For this review, take the finished solid that the model builds, in its own axes (mm). A direction names the side the tool comes from. Give positions to 0.01 mm unless a question says otherwise; leave off trailing zeros. Write each loop counter-clockwise with the first axis right and the second up, starting at its lowest first coordinate (ties: lowest second). Pieces come first, ordered by that corner, then holes. Notation, with made-up numbers: M 53,-37 L 76,-37 A34 ccw 76,2 Z; hole C 78.5,68 d10. An arc over 180 degrees is marked long. Use one line per item in the form item = value. Start each with the question number.
Q1. For probe 1 along Y at (x, z) = (-15.5, -8.25); probe 2 along Z at (x, y) = (26.75, -45); probe 3 along Y at (x, z) = (29.5, -11.5), list the stretches that pass through material, from the lowest coordinate up. Write a range as [from, to].
Q2. Consider section D-D on y = 30. Write out the cut boundary in (x, z), and give its area (3 significant figures).
Q3. Clearance check with flat-ended pins moving along their axes: pin 1 Ø3.5 at (y, z) = (-46, -7) entering from +X; pin 2 Ø3.5 at (y, z) = (39.5, -16.5) entering from -X; pin 3 Ø1 at (y, z) = (40.5, -16.5) entering from -X; pin 4 Ø6 at (x, z) = (-49, -12) entering from +Y. State where each tip first meets the part, or that it passes through.
Q4. Tool access review of faces 4 (the cylindrical face through (16.39, 41.39, -6.41)), 5 (the cylindrical face through (30.886, 47.003, -7.369)), 6 (the flat face through (-71.2, 9.44, -15.46)), 7 (the flat face through (-14, -1, -13)), 8 (the cylindrical face through (25.505, 0.22, -6.409)): name each direction out of +Z, -Z, +X, -X, +Y, -Y from which nothing blocks a thin tool from reaching the whole face with its end or side.
Q5. Mouldability with a two-part tool opening along X and no side actions: class faces 1 (the flat face through (21, -45, -8)), 2 (the flat face through (-18.25, 0, -16)), 3 (the cylindrical face through (30.886, 8.452, -6.581)) as released by +X, released by -X, zero draft, split by the parting line, or undercut.
Q6. Consider section A-A on x = 30.5. Give the number of separate pieces and of enclosed holes in the cut face, and give its area (3 significant figures).
Q7. Consider section B-B on x = -30.5. Write out the cut boundary in (y, z), and give its area (4 significant figures).
```python
from build123d import *

# Parameters (mm, degrees)
PAD_DEPTH       = 50
POCKET_DEPTH    = 18.001
SKETCH003_R     = 10.6
POCKET001_DEPTH = 30.4
SKETCH004_R     = 10.6
POCKET002_DEPTH = 30.4
SKETCH005_R     = 1.65
SKETCH005_R_2   = 2.65
POCKET007_DEPTH = 18.001
POCKET008_DEPTH = 5
SKETCH006_R     = 2.65
POCKET009_DEPTH = 18.001
SKETCH007_R     = 5
POCKET010_DEPTH = 13
SKETCH008_R     = 2.1
POCKET011_DEPTH = 20


with BuildPart() as part:
    # Sketch001 → Pad (new body, symmetric)
    with BuildSketch(Plane.XZ):
        with BuildLine():
            Line((-20.5, 0), (-6.5, 0))
            ThreePointArc((-6.5, 0), (0, -6.5), (6.5, 0))
            Line((6.5, 0), (20.5, 0))
            Line((20.5, 0), (40.5, 0))
            Line((40.5, 0), (40.5, -18))
            Line((40.5, -18), (20.5, -18))
            Line((20.5, -18), (-120.5, -18))
            Line((-120.5, -18), (-120.5, -13))
            Line((-20.5, -13), (-120.5, -13))
            Line((-20.5, 0), (-20.5, -13))
        make_face()
    extrude(amount=PAD_DEPTH, both=True)

    # Sketch002 → Pocket (cut, through all)
    with BuildSketch(Plane.XY):
        Polygon((-20.5, 50), (-120.5, 50), (-120.5, -30), align=None)
    extrude(amount=-POCKET_DEPTH, mode=Mode.SUBTRACT)

    # Sketch003 (on DatumPlane) → Pocket001 (cut)
    with BuildSketch(Plane.XZ.offset(45)):
        Circle(SKETCH003_R)
    extrude(amount=-POCKET001_DEPTH, mode=Mode.SUBTRACT)

    # Sketch004 (on DatumPlane) → Pocket002 (cut)
    with BuildSketch(Plane.XZ.offset(-45)):
        Circle(SKETCH004_R)
    extrude(amount=POCKET002_DEPTH, mode=Mode.SUBTRACT)

    # Sketch005 → Pocket007 (cut, through all)
    with BuildSketch(Plane.XY):
        with Locations((-15.5, -40)):
            Circle(SKETCH005_R)
        with Locations((15.5, -40)):
            Circle(SKETCH005_R)
        with Locations((15.5, 0)):
            Circle(SKETCH005_R)
        with Locations((15.5, 40)):
            Circle(SKETCH005_R)
        with Locations((-15.5, 40)):
            Circle(SKETCH005_R)
        with Locations((-15.5, 0)):
            Circle(SKETCH005_R)
        with Locations((-110.5, -40)):
            Circle(SKETCH005_R_2)
        with Locations((-70.5, -40)):
            Circle(SKETCH005_R_2)
        with Locations((-30.5, -40)):
            Circle(SKETCH005_R_2)
    extrude(amount=-POCKET007_DEPTH, mode=Mode.SUBTRACT)

    # Sketch (on DatumPlane) → Pocket008 (cut)
    with BuildSketch(Plane.XY.offset(-18)):
        Polygon((-12.75, 38.412287), (-12.75, 41.587713), (-15.5, 43.175426), (-18.25, 41.587713), (-18.25, 38.412287), (-15.5, 36.824574), align=None)
        Polygon((18.25, 38.412287), (18.25, 41.587713), (15.5, 43.175426), (12.75, 41.587713), (12.75, 38.412287), (15.5, 36.824574), align=None)
        Polygon((-12.75, -1.587713), (-12.75, 1.587713), (-15.5, 3.175426), (-18.25, 1.587713), (-18.25, -1.587713), (-15.5, -3.175426), align=None)
        Polygon((18.25, -1.587713), (18.25, 1.587713), (15.5, 3.175426), (12.75, 1.587713), (12.75, -1.587713), (15.5, -3.175426), align=None)
        Polygon((-12.75, -41.587713), (-12.75, -38.412287), (-15.5, -36.824574), (-18.25, -38.412287), (-18.25, -41.587713), (-15.5, -43.175426), align=None)
        Polygon((18.25, -41.587713), (18.25, -38.412287), (15.5, -36.824574), (12.75, -38.412287), (12.75, -41.587713), (15.5, -43.175426), align=None)
    extrude(amount=POCKET008_DEPTH, mode=Mode.SUBTRACT)

    # Sketch006 → Pocket009 (cut, through all)
    with BuildSketch(Plane.XY):
        with Locations((30.5, 40)):
            Circle(SKETCH006_R)
        with Locations((30.5, 0)):
            Circle(SKETCH006_R)
        with Locations((30.5, -40)):
            Circle(SKETCH006_R)
    extrude(amount=-POCKET009_DEPTH, mode=Mode.SUBTRACT)

    # Sketch007 → Pocket010 (cut)
    with BuildSketch(Plane.XY):
        with Locations((30.5, 40)):
            Circle(SKETCH007_R)
        with Locations((30.5, 0)):
            Circle(SKETCH007_R)
    extrude(amount=-POCKET010_DEPTH, mode=Mode.SUBTRACT)

    # Sketch008 (on DatumPlane) → Pocket011 (cut)
    with BuildSketch(Plane.YZ.offset(41)):
        with Locations((-45, -8)):
            Circle(SKETCH008_R)
        with Locations((-10, -8)):
            Circle(SKETCH008_R)
        with Locations((10, -8)):
            Circle(SKETCH008_R)
        with Locations((45, -8)):
            Circle(SKETCH008_R)
    extrude(amount=-POCKET011_DEPTH, mode=Mode.SUBTRACT)


solid = part.part
```
Working result:
q1.probe_1 = [-50, -41.65], [-38.35, -1.65], [1.65, 38.35], [41.65, 50]
q1.probe_2 = [-18, -10.1], [-5.9, 0]
q1.probe_3 = [-50, -42.45], [-37.55, -4.9], [4.9, 35.1], [44.9, 50]
q2.outline = M -45.5,-18 L 40.5,-18 L 40.5,0 L 10.6,0 A10.6 cw -10.6,0 L -20.5,0 L -20.5,-13 L -45.5,-13 Z
q2.area = 1,050 mm²
q3.pin_1 = 40.5
q3.pin_2 = -35.81
q3.pin_3 = -33
q3.pin_4 = 29.46
q4.face_4 = +Z, -Z
q4.face_5 = +X
q4.face_6 = +Z, -Z, -X, +Y
q4.face_7 = -Z
q4.face_8 = +Z
q5.face_1 = released by +X
q5.face_2 = undercut
q5.face_3 = zero draft
q6.separate_pieces = 4
q6.enclosed_holes = 3
q6.area = 1,340 mm²
q7.outline = M -50,-18 L -42.65,-18 L -42.65,-13 L -50,-13 Z; M -37.35,-18 L 42,-18 L 42,-13 L -37.35,-13 Z
q7.area = 433.5 mm²
